Design review of the part shown in the three views and the two pictorial views. Dimensions are in mm from the part's minimum x, y and z. A direction names the side the tool comes from. Coordinates: 2 decimals unless noted, no trailing zeros. Order: outer loops, then holes, each group sorted by start corner. A loop starts at its lowest first (then second) coordinate and runs counter-clockwise, first axis right, second up. Notation, with made-up numbers: (-11.75, 40.25) - (28.25, 40.25) arc R10 ccw to (28.25, 45.25) - close; hole circle Ø9 at (-30, 63). An arc over 180 degrees is marked (long way). One line per item, written item: value. Start each with the question number.
(1) To check wall thickness, follow line 1 along Y through (x, z) = (7, 21); line 2 along Z through (x, y) = (30, 10); line 3 along X through (y, z) = (11.75, 40.5). State the ranges of each line that lie inside material, in increasing order.
(2) Consider section D-D on z = 19. Write out the cut boundary in (x, y), then the cut area to 3 significant figures.
(3) For the marked faces 1, 2, 3 and 4, list the 3-axis set-ups (+Z, -Z, +X, -X, +Y, -Y) from which the entire face can be reached by the end or side of a thin tool; tool diameter is ignored.
(4) Consider section B-B on z = 25. Write out the cut boundary in (x, y).
(5) Consider section A-A on y = 10. Write out the cut boundary in (x, z) (3 decimals).
(6) Mouldability with a two-part tool opening along X and no side actions: class the marked faces 5, 6 and 7 as released by +X, released by -X, zero draft, split by the parting line, or undercut.
(7) Consider section C-C on x = 30. Write out the cut boundary in (y, z).
(8) Clearance check with flat-ended pins moving along their axes: pin 1 (4 mm diameter, centred on x = 54.5, y = 11, fed in from +Z); pin 2 (9 mm diameter, centred on x = 30, z = 25, fed in from -Y); pin 3 (4 mm diameter, centred on y = 5, z = 37, fed in from -X); pin 4 (10.5 mm diameter, centred on x = 5, y = 6.5, fed in from +Z). State where each tip first meets the part, or that it passes through.
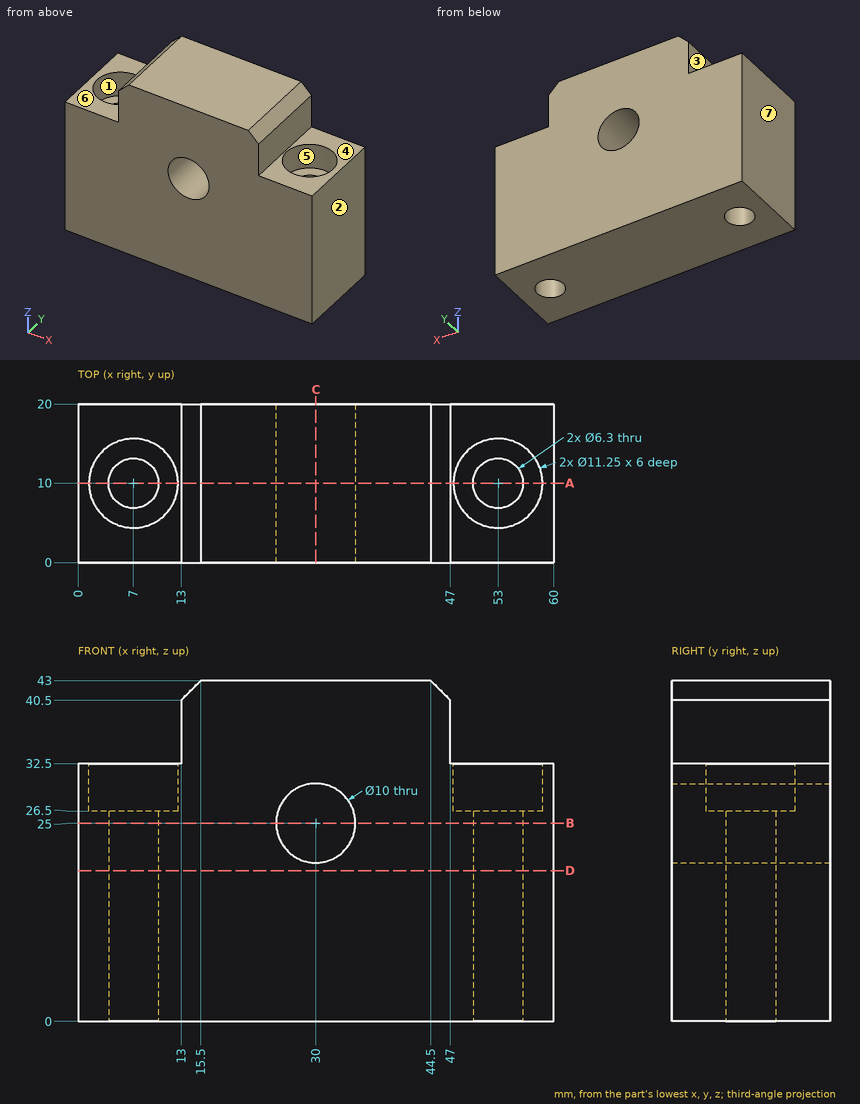
Geometry check:
1. line 1: y = 0 to 6.85, 13.15 to 20
1. line 2: z = 0 to 20, 30 to 43
1. line 3: x = 13 to 47
2. outline: (0, 0) - (60, 0) - (60, 20) - (0, 20) - close; hole circle Ø6.3 at (7, 10); hole circle Ø6.3 at (53, 10)
2. area: 1,140 mm^2
3. face 1: +Z
3. face 2: +Z, -Z, +X, +Y, -Y
3. face 3: +Z, -X, +Y, -Y
3. face 4: +Z, +X, +Y, -Y
4. outline: (0, 0) - (25, 0) - (25, 20) - (0, 20) - close; (35, 0) - (60, 0) - (60, 20) - (35, 20) - close; hole circle Ø6.3 at (7, 10); hole circle Ø6.3 at (53, 10)
5. outline: (0, 0) - (3.85, 0) - (3.85, 26.5) - (1.375, 26.5) - (1.375, 32.5) - (0, 32.5) - close; (10.15, 0) - (49.85, 0) - (49.85, 26.5) - (47.375, 26.5) - (47.375, 32.5) - (47, 32.5) - (47, 40.5) - (44.5, 43) - (15.5, 43) - (13, 40.5) - (13, 32.5) - (12.625, 32.5) - (12.625, 26.5) - (10.15, 26.5) - close; (56.15, 0) - (60, 0) - (60, 32.5) - (58.625, 32.5) - (58.625, 26.5) - (56.15, 26.5) - close; hole circle Ø10 at (30, 25)
6. face 5: undercut
6. face 6: zero draft
6. face 7: released by -X
7. outline: (0, 0) - (20, 0) - (20, 20) - (0, 20) - close; (0, 30) - (20, 30) - (20, 43) - (0, 43) - close
8. pin 1: stops at z = 26.5
8. pin 2: passes through
8. pin 3: stops at x = 13
8. pin 4: stops at z = 32.5
